Verification items for the finished model (mm, model axes). Face numbers are marked on the shaded views. Round coordinates to 2 decimals unless told otherwise and drop trailing zeros. Order: outer loops, then holes, each group sorted by start corner. A loop starts at its lowest first (then second) coordinate and runs counter-clockwise, first axis right, second up. Notation, with made-up numbers: (69.25, 67.25) -> (102.25, 67.25) arc R18 cw to (102.25, 95.25) -> close; hole circle Ø2 at (21.5, -28). An arc over 180 degrees is marked (long way). Answer in a Markdown table with one row per item. Add a question column.
Autodesk Inventor part; units mm, degrees
ref_plane "YZ Plane" through (0, 0, 0) normal (1, 0, 0) x (0, 1, 0)
ref_plane "XZ Plane" through (0, 0, 0) normal (0, 1, 0) x (-1, 0, 0)
ref_plane "XY Plane" through (0, 0, 0) normal (0, 0, 1) x (1, 0, 0)
ref_plane "Work Plane1" through (56.2325, -3.9241, -54.643) normal (0.9843, -0.1766, 0) x (0.1766, 0.9843, 0)
sketch "Sketch1" plane through (56.2325, -3.9241, -54.643) normal (0.9843, -0.1766, 0) x (0.1766, 0.9843, 0)
  line L0 (8.8813, -28.7707) -> (8.8813, -26.2307) construction
  line L1 (8.8813, -26.2307) -> (11.7241, -26.2307) construction
  line L2 (11.7241, -26.2307) -> (11.7241, -28.7707) construction
  line L3 (11.7241, -28.7707) -> (8.8813, -28.7707) construction
  line L4 (4.5958, -26.2307) -> (4.5958, -28.7707) construction
  line L5 (4.5958, -28.7707) -> (-5.2462, -28.7707) construction
  line L6 (-5.2462, -28.7707) -> (-5.2462, -26.2307) construction
  line L7 (-5.2462, -26.2307) -> (4.5958, -26.2307) construction
  line L8 (19.4818, -26.2307) -> (19.4818, -28.7707) construction
  line L9 (19.4818, -28.7707) -> (16.7961, -28.7707) construction
  line L10 (16.7961, -28.7707) -> (16.7961, -26.2307) construction
  line L11 (16.7961, -26.2307) -> (19.4818, -26.2307) construction
  spline S0 degree 2 poles (40.7352, 49.563) (36.4181, 6.3217) (32.911, -28.7707) knots 0 0 0 7.872352 7.872352 7.872352 weights 1 1.005429 1 construction
  line L12 (32.911, -28.7707) -> (24.0815, -28.7707) construction
  line L13 (24.0815, -28.7707) -> (24.0815, -26.2307) construction
  line L14 (24.0815, -26.2307) -> (30.6156, -26.2307) construction
  spline S1 degree 2 poles (30.6156, -26.2307) (33.9974, 7.5872) (38.19, 49.563) knots 0 0 0 7.617126 7.617126 7.617126 weights 1 1.005811 1 construction
  line L15 (38.19, 49.563) -> (38.4437, 52.103) construction
  line L16 (38.4437, 52.103) -> (48.6252, 52.103) construction
  line L17 (48.6252, 52.103) -> (48.6252, 43.213) construction
  line L18 (48.6252, 43.213) -> (46.0815, 43.213) construction
  line L19 (46.0815, 43.213) -> (46.0815, 49.563) construction
  line L20 (46.0815, 49.563) -> (40.7352, 49.563) construction
  spline S2 degree 2 poles (-34.4769, -28.7707) (-37.984, 6.3217) (-42.3012, 49.563) knots 0 0 0 7.872352 7.872352 7.872352 weights 1 1.005429 1 construction
  line L21 (-42.3012, 49.563) -> (-47.6475, 49.563) construction
  line L22 (-47.6475, 49.563) -> (-47.6475, 43.213) construction
  line L23 (-47.6475, 43.213) -> (-50.1911, 43.213) construction
  line L24 (-50.1911, 43.213) -> (-50.1911, 52.103) construction
  line L25 (-50.1911, 52.103) -> (-40.0096, 52.103) construction
  line L26 (-40.0096, 52.103) -> (-39.7559, 49.563) construction
  spline S3 degree 2 poles (-39.7559, 49.563) (-35.5633, 7.5872) (-32.1815, -26.2307) knots 0 0 0 7.617126 7.617126 7.617126 weights 1 1.005811 1 construction
  line L27 (-32.1815, -26.2307) -> (-8.6835, -26.2307) construction
  line L28 (-8.6835, -26.2307) -> (-8.6835, -28.7707) construction
  line L29 (-8.6835, -28.7707) -> (-34.4769, -28.7707) construction
  line L30 (43.5344, 52.103) -> (43.5344, 57.183)
  line L31 (43.5344, 52.103) -> (40.9944, 52.103)
  line L32 (40.9944, 52.103) -> (40.9944, 54.643)
  line L33 (40.9944, 54.643) -> (35.9144, 54.643)
  line L34 (35.9144, 54.643) -> (35.9144, 26.7834)
  line L35 (35.9144, 26.7834) -> (33.3744, 26.7834)
  line L36 (33.3744, 26.7834) -> (33.3744, 54.643)
  line L37 (33.3744, 54.643) -> (0, 54.643)
  line L38 (0, 57.183) -> (43.5344, 57.183)
  line L39 (0, 57.183) -> (0, 54.643)
  point P0 (-6.0665, 54.643)
  dimension "d1" = 5.08
  dimension "d4" = 2.54
  dimension "d5" = 2.54
  dimension "d6" = 5.08
  dimension "d7" = 2.54
  dimension "d8" = 2.54
  dimension "d9" = 48.6252
revolve "Revolution1" add sketch "Sketch1" angle 360 about axis through (56.2325, -3.9241, 2.54) along (0, 0, -1)
properties part number "lid" material "Stainless Steel"
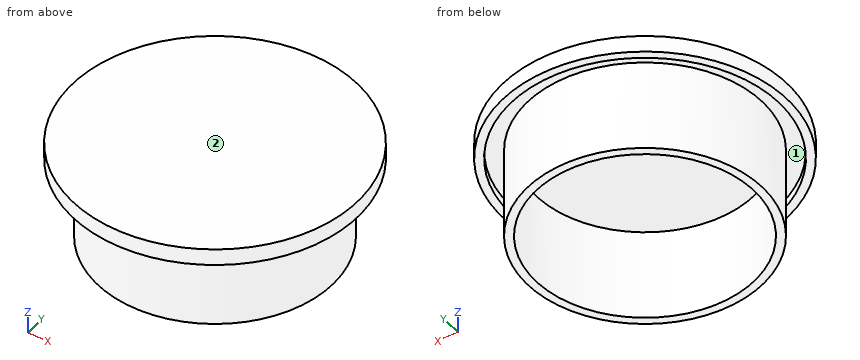
1) Depth check by flat-ended pin: P1, Ø8, axis at y = 10, z = -16, coming from the +X side; P2, Ø10, axis at x = 60.5, z = -22, coming from the -Y side; P3, Ø6, axis at y = 12.5, z = -17, coming from the +X side. Enter the tip coordinate at first touch or a pass-through.
2) Thickness scan on L1, parallel to Y at x = 49, z = -0.5; L2, parallel to Y at x = 56.5, z = -1.5; L3, parallel to Z at x = 66, y = -42. Record the ranges inside material, lowest first. Write a range as [from, to].
3) Cross-section at B-B, the plane y = 25. Record the boundary of the cut face in (x, z).
4) Draft check along X on the marked faces 1 and 2. Enter one of: +X half, -X half, draft (parallel to the pull), parting line (faces both ways), or undercut.
5) Cross-section at C-C, the plane z = -11.5. Record the boundary of the cut face in (x, y).
6) Cross-section at A-A, the plane x = 65. Record the boundary of the cut face in (y, z), and give its area (3 significant figures).
Results below:
| question | item | result |
|---|---|---|
| 1 | P1 | x = 90.75 |
| 1 | P2 | y = -39.84 |
| 1 | P3 | x = 89.54 |
| 2 | L1 | [-46.85, -44.28], [-39.1, -36.51], [28.66, 31.25], [36.43, 39.01] |
| 2 | L2 | [-47.46, -44.92], [-39.84, -37.3], [29.45, 31.99], [37.07, 39.61] |
| 2 | L3 | [0, 2.54] |
| 3 | outline | (23.7, -2.54) -> (27.18, -2.54) -> (27.18, 0) -> (34.94, 0) -> (34.94, -27.86) -> (39.58, -27.86) -> (39.58, 0) -> (72.88, 0) -> (72.88, -27.86) -> (77.52, -27.86) -> (77.52, 0) -> (85.28, 0) -> (85.28, -2.54) -> (88.77, -2.54) -> (88.77, 2.54) -> (23.7, 2.54) -> close |
| 4 | face 1 | undercut |
| 4 | face 2 | draft |
| 5 | outline | circle Ø71.83 at (56.23, -3.92); hole circle Ø66.75 at (56.23, -3.92) |
| 6 | outline | (-46.57, -2.54) -> (-43.97, -2.54) -> (-43.97, 0) -> (-38.75, 0) -> (-38.75, -27.86) -> (-36.13, -27.86) -> (-36.13, 0) -> (28.28, 0) -> (28.28, -27.86) -> (30.9, -27.86) -> (30.9, 0) -> (36.12, 0) -> (36.12, -2.54) -> (38.72, -2.54) -> (38.72, 2.54) -> (-46.57, 2.54) -> close |
| 6 | area | 376 mm² |
